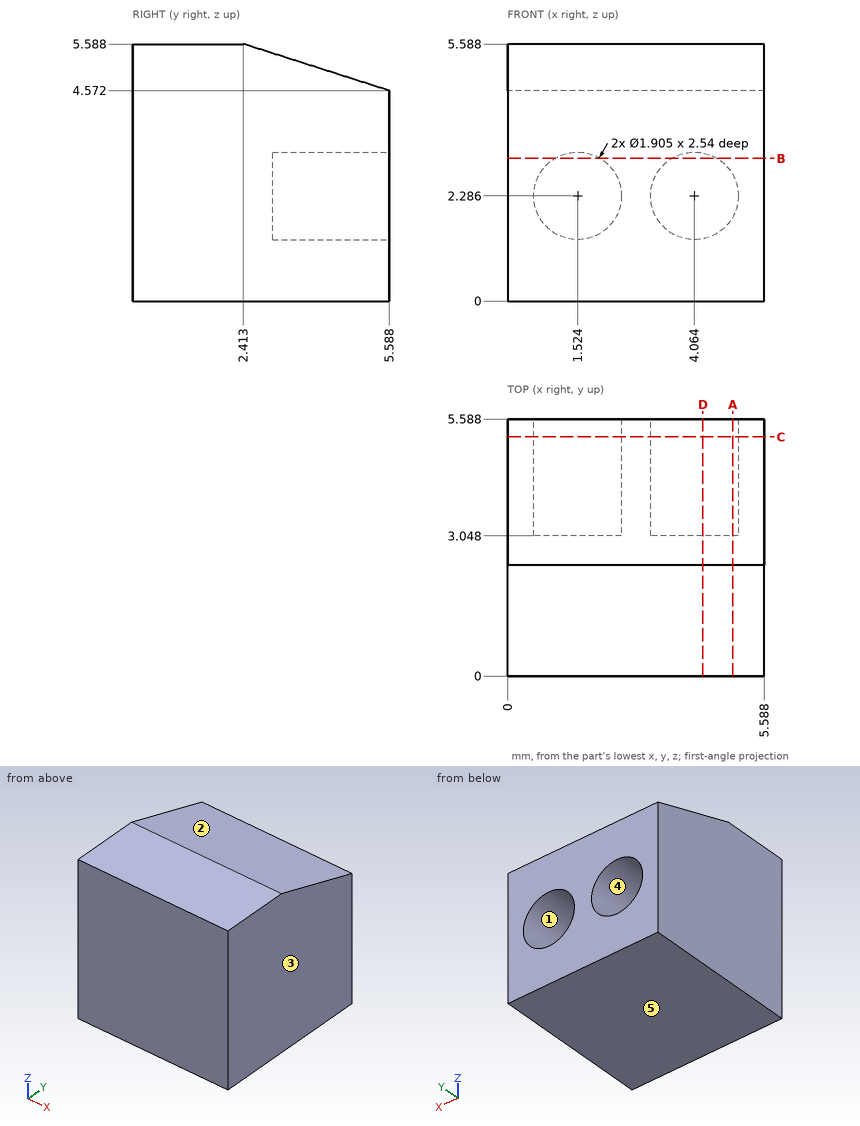
The figure shows three views and two pictorial views of one solid part (mm, origin at its lowest corner). Answer the questions. A direction names the side the tool comes from. Round coordinates to 2 decimals unless told otherwise and drop trailing zeros. Order: outer loops, then holes, each group sorted by start corner. A loop starts at its lowest first (then second) coordinate and runs counter-clockwise, first axis right, second up. Notation, with made-up numbers: (49, 80.25) - (83, 80.25) arc R15 ccw to (83, 103.25) - close; hole circle Ø2 at (-3.75, -39). An arc over 180 degrees is marked (long way). Write item = value, one per line. Start each with the question number.
1) Section A-A, the plane x = 4.9 is taken. Write down the section's boundary in (y, z).
2) Straight lines are drawn through the part: L1, parallel to X at y = 5.1, z = 2.85; L2, parallel to X at y = 3.9, z = 2.5; L3, parallel to Y at x = 4.3, z = 1.7. For each, find the intervals that lie inside material, in ascending order.
3) Section B-B, the plane z = 3.1 is taken. Write down the section's boundary in (x, y).
4) Given pin 1 (1 mm diameter, centred on x = 2.5, y = 4, fed in from +Z); pin 2 (0.6 mm diameter, centred on x = 4, z = 2.5, fed in from +Y), each flat-ended and moving along its own axis, determine where each tip first touches the part or whether it passes through.
5) Section C-C, the plane y = 5.2 is taken. Write down the section's boundary in (x, z) (1 decimal), plus the area to 3 significant figures.
6) For a pull along Z with two mould halves and no side action, classify the marked faces 3, 4 and 5 as released by +Z, released by -Z, zero draft, split by the parting line, or undercut.
7) Section D-D, the plane x = 4.25 is taken. Write down the section's boundary in (y, z), plus the area to 3 significant figures.
8) For the marked faces 1 and 2, determine the directions among +Z, -Z, +X, -X, +Y, -Y from which every point of the face is accessible in a straight line to the end or side of a thin tool.
Results list:
q1.outline = (0, 0) - (5.59, 0) - (5.59, 1.83) - (3.05, 1.83) - (3.05, 2.74) - (5.59, 2.74) - (5.59, 4.57) - (2.41, 5.59) - (0, 5.59) - close
q2.L1 = 0 to 0.76, 2.29 to 3.3, 4.83 to 5.59
q2.L2 = 0 to 0.6, 2.45 to 3.14, 4.99 to 5.59
q2.L3 = 0 to 3.05
q3.outline = (0, 0) - (5.59, 0) - (5.59, 5.59) - (4.56, 5.59) - (4.56, 3.05) - (3.57, 3.05) - (3.57, 5.59) - (2.02, 5.59) - (2.02, 3.05) - (1.03, 3.05) - (1.03, 5.59) - (0, 5.59) - close
q4.pin_1 = 5.24
q4.pin_2 = 3.05
q5.outline = (0, 0) - (5.6, 0) - (5.6, 4.7) - (0, 4.7) - close; hole circle Ø1.9 at (1.5, 2.3); hole circle Ø1.9 at (4.1, 2.3)
q5.area = 20.5 mm^2
q6.face_3 = zero draft
q6.face_4 = undercut
q6.face_5 = released by -Z
q7.outline = (0, 0) - (5.59, 0) - (5.59, 1.35) - (3.05, 1.35) - (3.05, 3.22) - (5.59, 3.22) - (5.59, 4.57) - (2.41, 5.59) - (0, 5.59) - close
q7.area = 24.9 mm^2
q8.face_1 = +Y
q8.face_2 = +Z, +X, -X, +Y
